from build123d import *

# Parameters (mm, degrees)
BOSS_EXTRUDE1_DEPTH = 4
SKETCH4_W           = 130
SKETCH4_H           = 4
BOSS_EXTRUDE2_DEPTH = 10
SKETCH5_W           = 130
SKETCH5_H           = 4
BOSS_EXTRUDE3_DEPTH = 7
SKETCH6_W           = 130
SKETCH6_H           = 4
BOSS_EXTRUDE4_DEPTH = 10
SKETCH7_W           = 130
SKETCH7_H           = 4
BOSS_EXTRUDE5_DEPTH = 7


with BuildPart() as part:
    # Sketch3 → Boss-Extrude1 (new body)
    with BuildSketch(Plane(origin=(0, 0, 0), x_dir=(1, 0, 0), z_dir=(0, 1, 0))):
        Polygon((-25, 80), (25, 80), (25, 76), (65, 76), (65, 25), (69, 25), (69, -25), (65, -25), (65, -76), (25, -76), (25, -80), (-25, -80), (-25, -76), (-65, -76), (-65, -25), (-69, -25), (-69, 25), (-65, 25), (-65, 76), (-25, 76), align=None)
    extrude(amount=BOSS_EXTRUDE1_DEPTH)

    # Sketch4 → Boss-Extrude2 (add)
    with BuildSketch(Plane(origin=(0, 4, 0), x_dir=(1, 0, 0), z_dir=(0, 1, 0))):
        with Locations((0, -74)):
            Rectangle(SKETCH4_W, SKETCH4_H)
    extrude(amount=BOSS_EXTRUDE2_DEPTH)

    # Sketch5 → Boss-Extrude3 (add)
    with BuildSketch(Plane(origin=(0, 4, 0), x_dir=(1, 0, 0), z_dir=(0, 1, 0))):
        with Locations((0, -66)):
            Rectangle(SKETCH5_W, SKETCH5_H)
    extrude(amount=BOSS_EXTRUDE3_DEPTH)

    # Sketch6 → Boss-Extrude4 (add)
    with BuildSketch(Plane(origin=(0, 4, 0), x_dir=(1, 0, 0), z_dir=(0, 1, 0))):
        with Locations((0, -6)):
            Rectangle(SKETCH6_W, SKETCH6_H)
    extrude(amount=BOSS_EXTRUDE4_DEPTH)

    # Sketch7 → Boss-Extrude5 (add)
    with BuildSketch(Plane(origin=(0, 4, 0), x_dir=(1, 0, 0), z_dir=(0, 1, 0))):
        with Locations((0, 2)):
            Rectangle(SKETCH7_W, SKETCH7_H)
    extrude(amount=BOSS_EXTRUDE5_DEPTH)


solid = part.part
Could you check a few things on this model? Use its own coordinates, in mm. A direction names the side the tool comes from. Give positions to 0.01 mm unless a question says otherwise; leave off trailing zeros. Order: outer loops, then holes, each group sorted by start corner. A loop starts at its lowest first (then second) coordinate and runs counter-clockwise, first axis right, second up. Notation, with made-up numbers: (85, -14.5) -> (120, -14.5) arc R12 ccw to (120, 3.5) -> close; hole circle Ø1 at (-33, 39). An arc over 180 degrees is marked (long way). Answer in a Markdown table with one row per item. Add a question column.
Item 1: For faces 1 (the flat face through (-1, 9, 4)), 2 (the flat face through (25, 2, 78)), 3 (the flat face through (67, 2, -25)), 4 (the flat face through (-65, 7, -2)), which set-ups out of +Z, -Z, +X, -X, +Y, -Y let a thin tool reach every point of the face, with its end or its side?
Item 2: Imagine slicing it at A-A (y = 5.75). List the corners of the cut face in (x, z) for me.
Item 3: Imagine slicing it at B-B (x = 20). List the corners of the cut face in (y, z) for me, and give its area (3 significant figures).
Item 4: I'm going to push flat-ended pins straight in: P1, Ø5.5, axis at x = 0.5, y = 7, coming from the +Z side; P2, Ø1.2, axis at x = 14, z = 70, coming from the +Y side; P3, Ø4.5, axis at y = 7, z = 6.5, coming from the +X side. Where does each tip first touch, or does it pass through?
Item 5: Please list where these lines run through material, in increasing order: probe 1 along Z at (x, y) = (-44, 6.5); probe 2 along Z at (x, y) = (-38.5, 12.25); probe 3 along X at (y, z) = (2.5, -66).
Item 6: Imagine slicing it at C-C (z = 21.5). List the corners of the cut face in (x, y) for me, and give its area (3 significant figures).
Item 7: Imagine slicing it at D-D (x = -45). List the corners of the cut face in (y, z) for me, and give its area (3 significant figures).
Result:
| question | item | result |
|---|---|---|
| 1 | face 1 | +X, -X, +Y |
| 1 | face 2 | +Z, +X, +Y, -Y |
| 1 | face 3 | -Z, +X, +Y, -Y |
| 1 | face 4 | +Z, -Z, -X, +Y |
| 2 | outline | (-65, -4) -> (65, -4) -> (65, 0) -> (-65, 0) -> close; (-65, 4) -> (65, 4) -> (65, 8) -> (-65, 8) -> close; (-65, 64) -> (65, 64) -> (65, 68) -> (-65, 68) -> close; (-65, 72) -> (65, 72) -> (65, 76) -> (-65, 76) -> close |
| 3 | outline | (0, -80) -> (4, -80) -> (4, -4) -> (11, -4) -> (11, 0) -> (4, 0) -> (4, 4) -> (14, 4) -> (14, 8) -> (4, 8) -> (4, 64) -> (11, 64) -> (11, 68) -> (4, 68) -> (4, 72) -> (14, 72) -> (14, 76) -> (4, 76) -> (4, 80) -> (0, 80) -> close |
| 3 | area | 776 mm2 |
| 4 | P1 | z = 76 |
| 4 | P2 | y = 4 |
| 4 | P3 | x = 65 |
| 5 | probe 1 | -4 to 0, 4 to 8, 64 to 68, 72 to 76 |
| 5 | probe 2 | 4 to 8, 72 to 76 |
| 5 | probe 3 | -65 to 65 |
| 6 | outline | (-69, 0) -> (69, 0) -> (69, 4) -> (-69, 4) -> close |
| 6 | area | 552 mm2 |
| 7 | outline | (0, -76) -> (4, -76) -> (4, -4) -> (11, -4) -> (11, 0) -> (4, 0) -> (4, 4) -> (14, 4) -> (14, 8) -> (4, 8) -> (4, 64) -> (11, 64) -> (11, 68) -> (4, 68) -> (4, 72) -> (14, 72) -> (14, 76) -> (0, 76) -> close |
| 7 | area | 744 mm2 |
